from build123d import *

# Parameters (mm, degrees)
SKETCH_W        = 104
SKETCH_H        = 62
PAD_DEPTH       = 20
SKETCH001_W     = 99
SKETCH001_H     = 57
POCKET_DEPTH    = 19
SKETCH002_W     = 6
SKETCH002_H     = 7
SKETCH002_R     = 1.2
PAD001_DEPTH    = 4
SKETCH003_W     = 75
SKETCH003_H     = 52
POCKET001_DEPTH = 1
SKETCH004_W     = 101.5
SKETCH004_H     = 59.5
SKETCH004_W_2   = 99
SKETCH004_H_2   = 57
PAD002_DEPTH    = 4
SKETCH005_W     = 0.5
SKETCH005_H     = 1.5
PAD003_DEPTH    = 50
FILLET_R        = 0.45
FILLET001_R     = 0.45
FILLET002_R     = 1
CHAMFER_SIZE    = 0.75
CHAMFER001_SIZE = 0.75
SKETCH006_W     = 8
SKETCH006_H     = 3
SKETCH006_H_2   = 4.5
POCKET002_DEPTH = 2.5
SKETCH009_W     = 13
SKETCH009_H     = 6.7
POCKET003_DEPTH = 1


with BuildPart() as part:
    # Sketch → Pad (new body)
    with BuildSketch(Plane.XY):
        Rectangle(SKETCH_W, SKETCH_H)
    extrude(amount=PAD_DEPTH)

    # Sketch001 (on Face6 of Pad) → Pocket (cut)
    with BuildSketch(Plane.XY.offset(20)):
        Rectangle(SKETCH001_W, SKETCH001_H)
    extrude(amount=-POCKET_DEPTH, mode=Mode.SUBTRACT)

    # Sketch002 (on Face11 of Pocket) → Pad001 (join)
    with BuildSketch(Plane.XY.offset(1)):
        with Locations((-46.5, 25)):
            Rectangle(SKETCH002_W, SKETCH002_H)
        with Locations((-46, 24.75)):
            Circle(SKETCH002_R, mode=Mode.SUBTRACT)
        with Locations((46.5, 25)):
            Rectangle(SKETCH002_W, SKETCH002_H)
        with Locations((46, 24.75)):
            Circle(SKETCH002_R, mode=Mode.SUBTRACT)
        with Locations((-46.5, -25)):
            Rectangle(SKETCH002_W, SKETCH002_H)
        with Locations((-46, -24.75)):
            Circle(SKETCH002_R, mode=Mode.SUBTRACT)
        with Locations((46.5, -25)):
            Rectangle(SKETCH002_W, SKETCH002_H)
        with Locations((46, -24.75)):
            Circle(SKETCH002_R, mode=Mode.SUBTRACT)
    extrude(amount=PAD001_DEPTH)

    # Sketch003 (on Face13 of Pad001) → Pocket001 (cut)
    with BuildSketch(Plane.XY.offset(1)):
        with Locations((-1.5, 0)):
            Rectangle(SKETCH003_W, SKETCH003_H)
    extrude(amount=-POCKET001_DEPTH, mode=Mode.SUBTRACT)

    # Sketch004 (on Face5 of Pocket001) → Pad002 (join)
    with BuildSketch(Plane.XY.offset(20)):
        Rectangle(SKETCH004_W, SKETCH004_H)
        Rectangle(SKETCH004_W_2, SKETCH004_H_2, mode=Mode.SUBTRACT)
    extrude(amount=PAD002_DEPTH)

    # Sketch005 (on Face14 of Pad002) → Pad003 (join)
    with BuildSketch(Plane(origin=(-23.75, 0, 0), x_dir=(0, -1, 0), z_dir=(-1, 0, 0))):
        with Locations((-30, 22)):
            Rectangle(SKETCH005_W, SKETCH005_H)
        with Locations((30, 22)):
            Rectangle(SKETCH005_W, SKETCH005_H)
        Polygon((-28.5, 7), (-27.5, 7), (-28.5, 10), align=None)
        Polygon((28.5, 7), (28.5, 10), (27.5, 7), align=None)
    extrude(amount=-PAD003_DEPTH)

    # Fillet
    fillet_edges = [part.edges().sort_by_distance(p)[0] for p in [
        (1.25, -30.25, 22.75),
        (1.25, -30.25, 21.25),
    ]]
    fillet(fillet_edges, radius=FILLET_R)

    # Fillet001
    fillet001_edges = [part.edges().sort_by_distance(p)[0] for p in [
        (1.25, 30.25, 22.75),
        (1.25, 30.25, 21.25),
    ]]
    fillet(fillet001_edges, radius=FILLET001_R)

    # Fillet002
    fillet002_edges = [part.edges().sort_by_distance(p)[0] for p in [
        (-50.75, -29.75, 22),
        (-52, -31, 10),
        (-50.75, 29.75, 22),
        (-52, 31, 10),
        (50.75, 29.75, 22),
        (52, 31, 10),
        (50.75, -29.75, 22),
        (52, -31, 10),
    ]]
    fillet(fillet002_edges, radius=FILLET002_R)

    # Chamfer
    chamfer_edges = [part.edges().sort_by_distance(p)[0] for p in [
        (-52, 0, 0),
        (0, -31, 0),
        (52, 0, 0),
        (0, 31, 0),
    ]]
    chamfer(chamfer_edges, length=CHAMFER_SIZE)

    # Chamfer001
    chamfer001_edges = [part.edges().sort_by_distance(p)[0] for p in [
        (-39, 0, 0),
        (-1.5, -26, 0),
        (36, 0, 0),
        (-1.5, 26, 0),
    ]]
    chamfer(chamfer001_edges, length=CHAMFER001_SIZE)

    # Sketch006 (on Face2 of Pad003) → Pocket002 (cut)
    with BuildSketch(Plane(origin=(-52, 0, 0), x_dir=(0, -1, 0), z_dir=(-1, 0, 0))):
        with Locations((12, 12.8)):
            Rectangle(SKETCH006_W, SKETCH006_H)
        with Locations((1.5, 13.05)):
            Rectangle(SKETCH006_W, SKETCH006_H_2)
    extrude(amount=-POCKET002_DEPTH, mode=Mode.SUBTRACT)

    # Sketch009 (on Face40 of Pocket002) → Pocket003 (cut)
    with BuildSketch(Plane.YZ.offset(-49.5)):
        with Locations((-1, 13.05)):
            Rectangle(SKETCH009_W, SKETCH009_H)
    extrude(amount=-POCKET003_DEPTH, mode=Mode.SUBTRACT)


solid = part.part
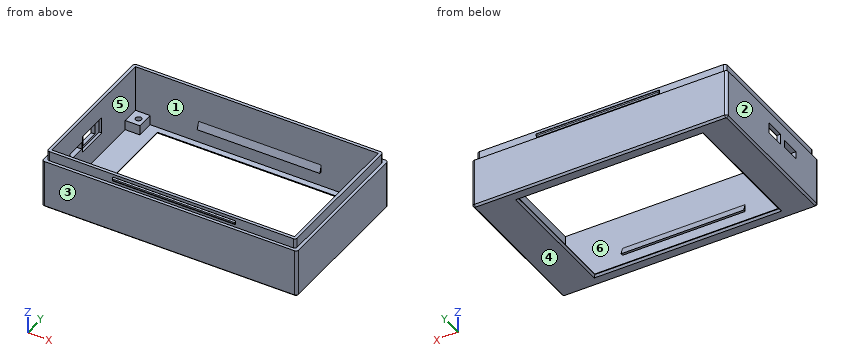
For this review, take the finished solid that the model builds, in its own axes (mm). Face numbers are marked on the shaded views. A direction names the side the tool comes from. Give positions to 0.01 mm unless a question says otherwise; leave off trailing zeros. Order: outer loops, then holes, each group sorted by start corner. A loop starts at its lowest first (then second) coordinate and runs counter-clockwise, first axis right, second up. Notation, with made-up numbers: (-18.75, -38) - (-1.75, -38) arc R24 cw to (-1.75, -21) - close; hole circle Ø8 at (33.5, 87). An arc over 180 degrees is marked (long way). Answer as a JSON object with one key per item and string values. Group by question number.
Item 1: Take a section at D-D on z = 3.75. Give the boundary of the cut face in (x, y).
Item 2: Wall thickness on line 1 along X through (y, z) = (-10, 18.75); line 2 along Y through (x, z) = (46, 1.8); line 3 along Y through (x, z) = (-7, 18.5): over which ranges is each line inside the solid? List them lowest first.
Item 3: Clearance check with flat-ended pins moving along their axes: pin 1 Ø0.8 at (x, z) = (-51.5, 12.5) entering from +Y (3 decimals); pin 2 Ø12 at (x, y) = (-11.5, 19) entering from -Z. State where each tip first meets the part, or that it passes through.
Item 4: Draft analysis for pull direction X (two halves, no side actions). For the marked faces 1, 2 and 3, state which applies: pulls with the +X half, pulls with the -X half, needs draft (parallel to the pull), parting line crosses it, or undercut.
Item 5: Take a section at A-A on z = 12.5. Give the boundary of the cut face in (x, y), and give its area (3 significant figures).
Item 6: Take a section at C-C on x = -38. Give the boundary of the cut face in (y, z), and give its area (3 significant figures).
Item 7: Machinability: for the marked faces 4, 5 and 6, which of the approach directions +Z, -Z, +X, -X, +Y, -Y give a long, thin tool a straight path to every point of the face, cutting with its end or side? Answer none if there is none.
Reported:
{
 "1": {"outline": "(-52, -30) arc R1 ccw to (-51, -31) - (51, -31) arc R1 ccw to (52, -30) - (52, 30) arc R1 ccw to (51, 31) - (-51, 31) arc R1 ccw to (-52, 30) - close; hole (-49.5, -21.5) - (-43.5, -21.5) - (-43.5, -28.5) - (43.5, -28.5) - (43.5, -21.5) - (49.5, -21.5) - (49.5, 21.5) - (43.5, 21.5) - (43.5, 28.5) - (-43.5, 28.5) - (-43.5, 21.5) - (-49.5, 21.5) - close; hole circle Ø2.4 at (-46, -24.75); hole circle Ø2.4 at (-46, 24.75); hole circle Ø2.4 at (46, -24.75); hole circle Ø2.4 at (46, 24.75)"},
 "2": {"line 1": "-52 to -49.5, 49.5 to 52", "line 2": "-31 to -25.95, -23.55 to -21.5, 21.5 to 23.55, 25.95 to 31", "line 3": "-31 to -28.5, 28.5 to 31"},
 "3": {"pin 1": "y = 30.995", "pin 2": "through"},
 "4": {"face 1": "undercut", "face 2": "pulls with the -X half", "face 3": "needs draft"},
 "5": {"outline": "(-52, -30) arc R1 ccw to (-51, -31) - (51, -31) arc R1 ccw to (52, -30) - (52, 30) arc R1 ccw to (51, 31) - (-51, 31) arc R1 ccw to (-52, 30) - (-52, 2.5) - (-50.5, 2.5) - (-50.5, 5.5) - (-49.5, 5.5) - (-49.5, 28.5) - (49.5, 28.5) - (49.5, -28.5) - (-49.5, -28.5) - (-49.5, -16) - (-52, -16) - close; (-52, -8) - (-49.5, -8) - (-49.5, -7.5) - (-50.5, -7.5) - (-50.5, -5.5) - (-52, -5.5) - close", "area": "759 mm^2"},
 "6": {"outline": "(-31, 0.75) - (-30.25, 0) - (-26.75, 0) - (-26, 0.75) - (-26, 1) - (-28.5, 1) - (-28.5, 24) - (-29.75, 24) - (-29.75, 20) - (-31, 20) - close; (26, 0.75) - (26.75, 0) - (30.25, 0) - (31, 0.75) - (31, 20) - (29.75, 20) - (29.75, 24) - (28.5, 24) - (28.5, 1) - (26, 1) - close", "area": "114 mm^2"},
 "7": {"face 4": "-Z, +X, -X, +Y, -Y", "face 5": "+Z", "face 6": "none"}
}
